Source: CAD feature listing. Evaluate the final solid. Frame: model axes, mm. Face numbers are marked on the shaded views. A direction names the side the tool comes from. Give positions to 0.01 mm unless a question says otherwise; leave off trailing zeros. Loops run counter-clockwise (first coordinate to the right, second up) from the corner with the lowest first, then second, coordinate; pieces in that order, holes last. Notation, with made-up numbers: (-12, 65.25) - (2, 65.25) arc R27 ccw to (2, 104.25) - close; hole circle Ø5 at (82, 50.5). An arc over 180 degrees is marked (long way). Write each question's results on one line, items separated by ' | '. Start each with the question number.
(1) Contact query for flat-ended pins moving along their axis: pin 1 (1 mm diameter, centred on x = 25, z = 52, fed in from -Y); pin 2 (8 mm diameter, centred on x = 35.5, y = 33, fed in from +Z) (3 decimals); pin 3 (8.5 mm diameter, centred on y = -16.5, z = 22.5, fed in from -X) (3 decimals). Output: stop coordinate, or through.
(2) Cut plane C-C on x = 70.5. Return the cut outline in (y, z) (3 decimals).
(3) Material intervals for line 1 along Y through (x, z) = (41, 18); line 2 along Z through (x, y) = (-26.5, 45.5) (3 decimals); line 3 along Y through (x, z) = (83, 46.5), sorted ascending. Write a range as [from, to].
(4) Cut plane B-B on x = 92. Return the cut outline in (y, z) (3 decimals).
(5) Reachability of the marked faces 1, 2, 3 and 4 from +Z, -Z, +X, -X, +Y, -Y: full face, straight path, thin tool, end or side. Return the list, or none.
(6) Cut plane A-A on z = 2. Return the cut outline in (x, y) (3 decimals), then the cut area to 3 significant figures.
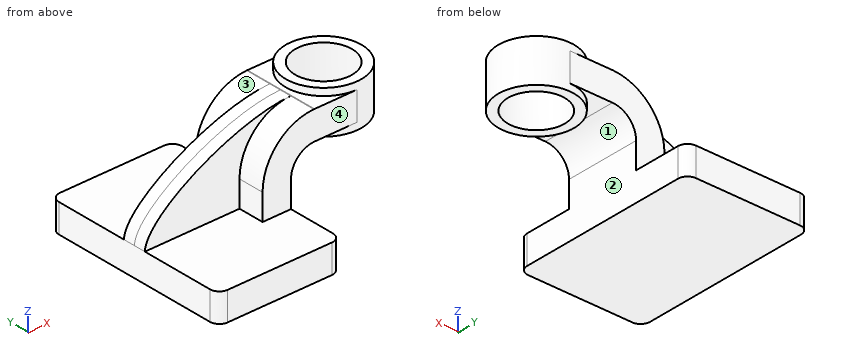
from build123d import *

# Parameters (mm, degrees)
F1_DEPTH = 63.5
F0_W     = 25.4
F0_H     = 19.05
F2_DEPTH = 25.4
F3_DEPTH = 7.9375
F5_R     = 6.35
F6_R     = 19.05
F7_DEPTH = 76.201


with BuildPart() as f1:
    # F0 (on Front) → F1 (new body, symmetric)
    with BuildSketch(Plane.XZ):
        Polygon((22.225, 9.525), (-41.275, 9.525), (-41.275, -9.525), (41.275, -9.525), (41.275, 9.525), align=None)
    extrude(amount=F1_DEPTH, both=True)

    # F0 (on Front) → F2 (join, symmetric)
    with BuildSketch(Plane.XZ):
        with Locations((73.025, 52.324)):
            Rectangle(F0_W, F0_H)
        with BuildLine():
            Line((22.225, 26.924), (22.225, 9.525))
            Line((22.225, 9.525), (41.275, 9.525))
            Line((41.275, 9.525), (41.275, 26.924))
            ThreePointArc((41.275, 26.924), (45.9246798487, 38.1493201513), (57.15, 42.799))
            Line((57.15, 42.799), (60.325, 42.799))
            Line((60.325, 42.799), (60.325, 61.849))
            Line((60.325, 61.849), (57.15, 61.849))
            add(Edge.make_bspline(
                [(56.5700312236, 61.8441841521), (56.7638831391, 61.8466038705), (56.957209462, 61.8482110704), (57.15, 61.849)],
                knots=[110.90829632, 110.90829632, 110.90829632, 110.90829632, 111.468747194, 111.468747194, 111.468747194, 111.468747194], degree=3))
            ThreePointArc((56.5700312236, 61.8441841521), (32.2500900151, 51.4137959923), (22.225, 26.924))
        make_face()
    extrude(amount=F2_DEPTH, both=True)

    # F0 (on Front) → F3 (join, symmetric)
    with BuildSketch(Plane.XZ):
        with BuildLine():
            add(Edge.make_bspline(
                [(-41.275, 9.525), (-40.7358347138, 29.0675254726), (18.2084429422, 61.3653431795), (56.5700312236, 61.8441841521)],
                knots=[0, 0, 0, 0, 110.90829632, 110.90829632, 110.90829632, 110.90829632], degree=3))
            Line((-41.275, 9.525), (22.225, 9.525))
            Line((22.225, 9.525), (22.225, 26.924))
            ThreePointArc((22.225, 26.924), (32.2500900151, 51.4137959923), (56.5700312236, 61.8441841521))
        make_face()
    extrude(amount=F3_DEPTH, both=True)

    # F0 (on Front) → F4 (revolve)
    with BuildSketch(Plane.XZ):
        Polygon((85.725, 66.675), (85.725, 61.849), (85.725, 42.799), (85.725, 38.1), (111.125, 38.1), (111.125, 66.675), align=None)
    revolve(axis=Axis((85.725, 0, 52.3875), (0, 0, 1)))

    # F5
    f5_edges = [f1.edges().sort_by_distance(p)[0] for p in [
        (41.275, -63.5, 0),
        (-41.275, -63.5, 0),
        (41.275, 63.5, 0),
        (-41.275, 63.5, 0),
    ]]
    fillet(f5_edges, radius=F5_R)

    # F6 (on face) → F7 (cut, through all)
    with BuildSketch(Plane.XY.offset(66.675)):
        with Locations((85.725, 0)):
            Circle(F6_R)
    extrude(amount=-F7_DEPTH, mode=Mode.SUBTRACT)


solid = f1.part
Ans:
1) pin 1: y = -7.94 | pin 2: z = 9.525 | pin 3: x = 22.225
2) outline: (-25.4, 42.799) - (-20.331, 42.799) - (-20.331, 38.1) - (-11.45, 38.1) - (-11.45, 66.675) - (-20.331, 66.675) - (-20.331, 61.849) - (-25.4, 61.849) - close; (11.45, 38.1) - (20.331, 38.1) - (20.331, 42.799) - (25.4, 42.799) - (25.4, 61.849) - (20.331, 61.849) - (20.331, 66.675) - (11.45, 66.675) - close
3) line 1: [-25.4, 25.4] | line 2: [-9.525, 9.525] | line 3: [-25.4, -18.85], [18.85, 25.4]
4) outline: (-24.613, 38.1) - (-17.987, 38.1) - (-17.987, 66.675) - (-24.613, 66.675) - close; (17.987, 38.1) - (24.613, 38.1) - (24.613, 66.675) - (17.987, 66.675) - close
5) face 1: -Z, +Y, -Y | face 2: -Z, +X, +Y, -Y | face 3: +Z, -X, +Y | face 4: +Z, +X, -X, -Y
6) outline: (-41.275, -57.15) arc R6.35 ccw to (-34.925, -63.5) - (34.925, -63.5) arc R6.35 ccw to (41.275, -57.15) - (41.275, 57.15) arc R6.35 ccw to (34.925, 63.5) - (-34.925, 63.5) arc R6.35 ccw to (-41.275, 57.15) - close | area: 10,400 mm^2
